Source: CAD feature listing. Evaluate the final solid. Frame: model axes, mm. A direction names the side the tool comes from. Give positions to 0.01 mm unless a question says otherwise; leave off trailing zeros. Order: outer loops, then holes, each group sorted by start corner. A loop starts at its lowest first (then second) coordinate and runs counter-clockwise, first axis right, second up. Notation, with made-up numbers: (74, -30.75) - (102, -30.75) arc R31 cw to (102, 1.25) - close; hole circle Ø6 at (44, 69). An arc over 180 degrees is marked (long way). Answer as CSV lines item,"result".
```python
from build123d import *

# Parameters (mm, degrees)
F0_W     = 15
F0_H     = 5
F1_DEPTH = 100
F2_W     = 5
F2_H     = 5
F3_DEPTH = 10
F4_W     = 5
F4_H     = 5
F5_DEPTH = 10
F6_DEPTH = 4
F7_R     = 2


with BuildPart() as f1:
    # F0 (on Right) → F1 (new body)
    with BuildSketch(Plane.YZ):
        with Locations((-8.0427642167, 0.8986243606)):
            Rectangle(F0_W, F0_H)
    extrude(amount=F1_DEPTH)

    # F2 (on face) → F3 (join)
    with BuildSketch(Plane.YZ.offset(100)):
        with Locations((-8.0427642167, 0.8986243606)):
            Rectangle(F2_W, F2_H)
    extrude(amount=F3_DEPTH)

    # F4 (on face) → F5 (join)
    with BuildSketch(Plane(origin=(0, 0, 0), x_dir=(0, -1, 0), z_dir=(-1, 0, 0))):
        with Locations((8.0427642167, 0.8986243606)):
            Rectangle(F4_W, F4_H)
    extrude(amount=F5_DEPTH)

    # F6 (cut): faces of the model
    f6_faces = [f1.faces().sort_by_distance(p)[0] for p in [
        (100, -13.0427642167, 0.8986243606),
        (100, -3.0427642167, 0.8986243606),
        (110, -8.0427642167, 0.8986243606),
    ]]
    extrude(f6_faces, amount=-F6_DEPTH, mode=Mode.SUBTRACT)

    # F7
    f7_edges = [f1.edges().sort_by_distance(p)[0] for p in [
        (48, -15.542764, 3.398624),
        (48, -0.542764, 3.398624),
        (48, -0.542764, -1.601376),
        (48, -15.542764, -1.601376),
    ]]
    fillet(f7_edges, radius=F7_R)


solid = f1.part
```
(1) Ray query, line 1 (Y direction, x = 30.5, z = 0.2); line 2 (Y direction, x = 98, z = 1.1); line 3 (X direction, y = -5.5, z = -0.3). Return the intervals inside material, ascending. Write a range as from..to.
Completed:
line 1,"-15.53..-0.55"
line 2,"-10.54..-5.54"
line 3,"0..96"
(2) Cut plane B-B (x = -3). Return loops of the section in (y, z), then the cut area to 3 significant figures.
Completed:
outline,"(-10.54, -1.6) - (-5.54, -1.6) - (-5.54, 3.4) - (-10.54, 3.4) - close"
area,"25.0 mm²"
(3) Cut plane A-A (x = 74). Return loops of the section in (y, z), then the cut area to 3 significant figures.
Completed:
outline,"(-15.54, 0.4) arc R2 ccw to (-13.54, -1.6) - (-2.54, -1.6) arc R2 ccw to (-0.54, 0.4) - (-0.54, 1.4) arc R2 ccw to (-2.54, 3.4) - (-13.54, 3.4) arc R2 ccw to (-15.54, 1.4) - close"
area,"71.6 mm²"
(4) Contact query for flat-ended pins moving along their axis: pin 1 (1.5 mm diameter, centred on x = -4, z = 0.5, fed in from +Y); pin 2 (2.5 mm diameter, centred on x = -6, z = 0, fed in from -Y); pin 3 (2.5 mm diameter, centred on y = -13, z = 0.5, fed in from +X). Output: stop coordinate, or through.
Completed:
pin 1,"y = -5.54"
pin 2,"y = -10.54"
pin 3,"x = 96"
(5) Access query for faces 1 (the flat face through (-5, -5.543, 1)), 2 (the flat face through (0, -13, 1)), 3 (the flat face through (96, -3, 1)), 4 (the flat face through (101, -10.543, 1)). Directions: +Z, -Z, +X, -X, +Y, -Y. A direction counts if a zero-diameter tool reaches every point of the face in a straight line with its end or side. Return the directions, or none.
Completed:
face 1,"+Z, -Z, -X, +Y"
face 2,"+Z, -Z, -X, -Y"
face 3,"+Z, -Z, +X, +Y"
face 4,"+Z, -Z, +X, -Y"
